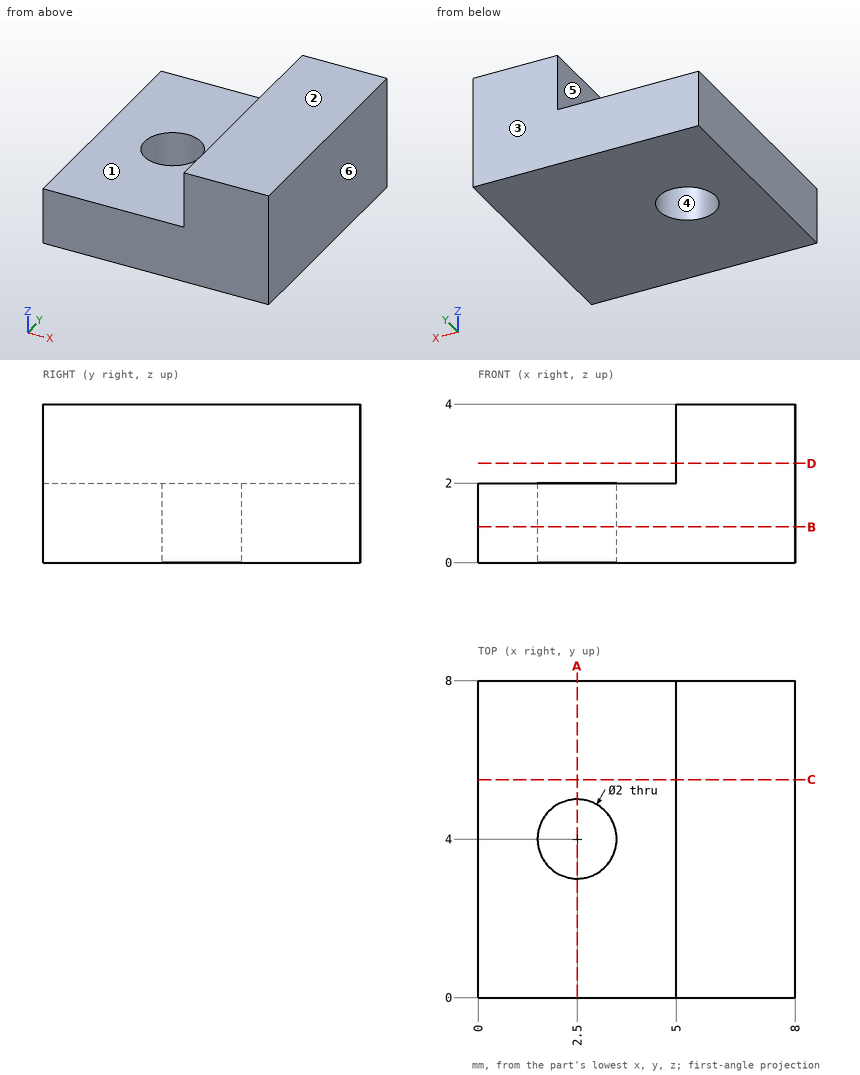
Part print with two shaded views. Sizes in mm from the minimum x, y, z corner. A direction names the side the tool comes from. Round coordinates to 2 decimals unless told otherwise and drop trailing zeros. Order: outer loops, then holes, each group sorted by start corner. A loop starts at its lowest first (then second) coordinate and runs counter-clockwise, first axis right, second up.
(1) Band-saw the part on C-C (y = 5.5). List the corners of the cut face in (x, z), then the cut area to 3 significant figures.
(2) Band-saw the part on B-B (z = 0.9). List the corners of the cut face in (x, y).
(3) 3-axis set-ups, long thin cutter, end or side, ignore diameter. For the marked faces 1 and 2: which of +Z, -Z, +X, -X, +Y, -Y reach the whole face in a straight line?
(4) Band-saw the part on D-D (z = 2.5). List the corners of the cut face in (x, y), then the cut area to 3 significant figures.
(5) Pull direction X, two halves, no side cores. Call the marked faces 3, 4, 5 and 6: released by +X, released by -X, zero draft, split by the parting line, or undercut.
(6) Pin check, flat tips, straight feed: pin 1 (1.2 mm diameter, centred on x = 2.5, y = 4, fed in from -Z); pin 2 (1 mm diameter, centred on x = 1, y = 4, fed in from +Z). Stop position of each tip, or through.
(7) Drill centre lines: line 1 (Y direction, x = 2.5, z = 1); line 2 (Z direction, x = 2.75, y = 6.75); line 3 (X direction, y = 4, z = 2.9). Where is each one in solid material? Low to high.
(8) Band-saw the part on A-A (x = 2.5). List the corners of the cut face in (y, z), then the cut area to 3 significant figures.
Verdict:
1. outline: (0, 0) - (8, 0) - (8, 4) - (5, 4) - (5, 2) - (0, 2) - close
1. area: 22.0 mm2
2. outline: (0, 0) - (8, 0) - (8, 8) - (0, 8) - close; hole circle Ø2 at (2.5, 4)
3. face 1: +Z, -X, +Y, -Y
3. face 2: +Z, +X, -X, +Y, -Y
4. outline: (5, 0) - (8, 0) - (8, 8) - (5, 8) - close
4. area: 24.0 mm2
5. face 3: zero draft
5. face 4: undercut
5. face 5: released by -X
5. face 6: released by +X
6. pin 1: passes through
6. pin 2: stops at z = 2
7. line 1: y = 0 to 3, 5 to 8
7. line 2: z = 0 to 2
7. line 3: x = 5 to 8
8. outline: (0, 0) - (3, 0) - (3, 2) - (0, 2) - close; (5, 0) - (8, 0) - (8, 2) - (5, 2) - close
8. area: 12.0 mm2
